Could you check a few things on this model? Use its own coordinates, in mm. A direction names the side the tool comes from. Round coordinates to 2 decimals unless told otherwise and drop trailing zeros. Write each loop counter-clockwise with the first axis right and the second up, starting at its lowest first coordinate (ties: lowest second). Pieces come first, ordered by that corner, then holes. Notation, with made-up numbers: M 4,66.25 L 14,66.25 A20 cw 14,87.25 Z; hole C 82.25,-19 d5. An arc over 180 degrees is marked long. One line per item, written item: value. Start each with the question number.
(1) Thinking about a two-plate mould opening in Y: for faces 3 (the face through (4, 20, 0)), 4 (the face through (6, 5, 1)), 5 (the face through (-0.195, -3.513, -0.084)), 6 (the face through (3.04, 4.98, -0.61)), which applies, released by +Y, released by -Y, zero draft, split by the parting line, or undercut?
(2) I want a section at D-D on x = 2.25. Please give me the cut outline in (y, z).
(3) I'm going to push flat-ended pins straight in: pin 1 Ø5.5 at (y, z) = (3, 2.5) entering from -X; pin 2 Ø6 at (y, z) = (11, 2.5) entering from -X; pin 3 Ø2.5 at (x, y) = (0, -5) entering from -Z; pin 4 Ø3 at (x, z) = (-2.5, -2.5) entering from +Y. Where does each tip first touch, or does it pass through?
(4) I want a section at A-A on z = 0. Please give me the cut outline in (x, y).
(5) I want a section at C-C on z = 2. Please give me the cut outline in (x, y).
(6) I want a section at B-B on y = -5. Please give me the cut outline in (x, z).
(7) If I drill on L1, parallel to X at y = 7.5, z = -4.75; L2, parallel to X at y = 0.75, z = 3.5; L3, parallel to Y at x = -4, z = -3, over which ranges is the centre line in solid material (lowest first)?
(8) Which directions (+Z, -Z, +X, -X, +Y, -Y) give clear straight access to the entire face, cutting with the end or side of a thin tool? Please do faces 1 (the face through (1, 2, -6)), 2 (the face through (0, 5, 1)).
```python
from build123d import *

# Parameters (mm, degrees)
F0_R     = 1.5
F1_DEPTH = 6
F4_DEPTH = 25


with BuildPart() as f1:
    # F0 (on Top) → F1 (new body, symmetric)
    with BuildSketch(Plane.XY):
        Polygon((6, -10), (6, 20), (1, 20), (1, 7), (0, 7), (0, 0), (-6, 0), (-6, -10), align=None)
        with Locations((0, -5)):
            Circle(F0_R, mode=Mode.SUBTRACT)
    extrude(amount=F1_DEPTH, both=True)

    # F3 (on offset) → F4 (cut)
    with BuildSketch(Plane.YZ.offset(6)):
        with BuildLine():
            ThreePointArc((1.9, 0), (3.5, -1.6), (5.1, 0))
            ThreePointArc((5.1, 0), (3.5, 1.6), (1.9, 0))
        make_face()
    extrude(amount=-F4_DEPTH, mode=Mode.SUBTRACT)


solid = f1.part
```
Found:
1. face 3: released by +Y
1. face 4: zero draft
1. face 5: undercut
1. face 6: undercut
2. outline: M -10,-6 L 20,-6 L 20,6 L -10,6 Z; hole C 3.5,0 d3.2
3. pin 1: stops at x = 0
3. pin 2: stops at x = 1
3. pin 3: passes through
3. pin 4: stops at y = 0
4. outline: M -6,-10 L 6,-10 L 6,1.9 L 0,1.9 L 0,0 L -6,0 Z; M 0,5.1 L 6,5.1 L 6,20 L 1,20 L 1,7 L 0,7 Z; hole C 0,-5 d3
5. outline: M -6,-10 L 6,-10 L 6,20 L 1,20 L 1,7 L 0,7 L 0,0 L -6,0 Z; hole C 0,-5 d3
6. outline: M -6,-6 L -1.5,-6 L -1.5,6 L -6,6 Z; M 1.5,-6 L 6,-6 L 6,6 L 1.5,6 Z
7. L1: x = 1 to 6
7. L2: x = 0 to 6
7. L3: y = -10 to 0
8. face 1: -Z, +X, -X, +Y, -Y
8. face 2: +Z, -Z, -X, +Y
